Here's how the part is built. I have some questions about the finished solid (model axes, mm). Face numbers are marked on the shaded views. Give positions to 0.01 mm unless a question says otherwise; leave off trailing zeros. Write each loop counter-clockwise with the first axis right and the second up, starting at its lowest first coordinate (ties: lowest second). Pieces come first, ordered by that corner, then holes. Notation, with made-up numbers: M -38.5,23.25 L 4.5,23.25 A20 cw 4.5,41.25 Z; hole C 77.25,60.25 d7. An arc over 180 degrees is marked long. Answer as CSV lines item,"result". Start each with the question number.
Q1. Suppose I cut it at C-C (x = -790.5). Write out the boundary of the cut face in (y, z).
Q2. Suppose I cut it at B-B (z = 392). Write out the boundary of the cut face in (x, y).
Q3. If I drill on line 1 along Y through (x, z) = (55, 360.5); line 2 along Y through (x, z) = (481, 328.5); line 3 along X through (y, z) = (-389, 378.5), over which ranges is the centre line in solid material (lowest first)?
Q4. Thinking about a two-plate mould opening in Y: for the marked faces 1, 2, 3 and 4, which applies, +Y half, -Y half, draft (parallel to the pull), parting line (faces both ways), or undercut?
Q5. Suppose I cut it at A-A (y = 576). Write out the boundary of the cut face in (x, z), then the cut area to 3 significant figures.
Q6. For pin 1 (5 mm diameter, centred on x = -303.5, y = 399, fed in from +Z), with a flat end and sliding along its axis, tell me the tip position at first contact or that it passes through.
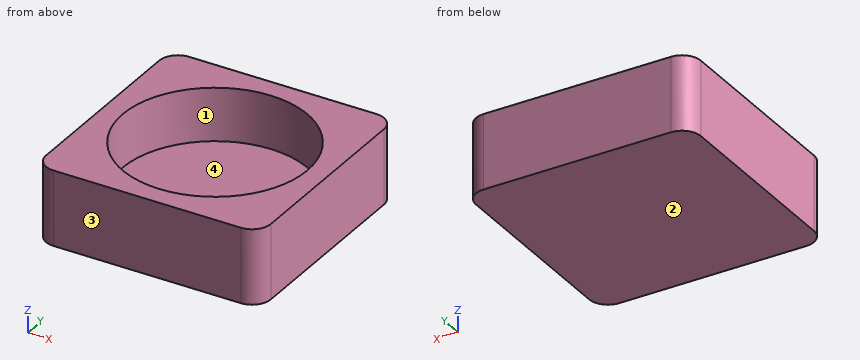
```python
from build123d import *

# Parameters (mm, degrees)
F0_W     = 1828.8
F0_H     = 1828.8
F1_DEPTH = 609.6
F2_R     = 751.405034
F3_DEPTH = 431.8
F4_R     = 152.4


with BuildPart() as f1:
    # F0 (on Top) → F1 (new body)
    with BuildSketch(Plane.XY):
        with Locations((-78.992321, -32.782064)):
            Rectangle(F0_W, F0_H)
    extrude(amount=F1_DEPTH)

    # F2 (on face) → F3 (cut)
    with BuildSketch(Plane.XY.offset(609.6)):
        with Locations((-78.992321, -32.782064)):
            Circle(F2_R)
    extrude(amount=-F3_DEPTH, mode=Mode.SUBTRACT)

    # F4
    f4_edges = [f1.edges().sort_by_distance(p)[0] for p in [
        (-993.392321, -947.182064, 304.8),
        (835.407679, -947.182064, 304.8),
        (835.407679, 881.617936, 304.8),
        (-993.392321, 881.617936, 304.8),
    ]]
    fillet(f4_edges, radius=F4_R)


solid = f1.part
```
Resolved:
1,outline,"M -947.18,0 L 881.62,0 L 881.62,609.6 L 208.81,609.6 L 208.81,177.8 L -274.37,177.8 L -274.37,609.6 L -947.18,609.6 Z"
2,outline,"M -993.39,-794.78 A152.4 ccw -840.99,-947.18 L 683.01,-947.18 A152.4 ccw 835.41,-794.78 L 835.41,729.22 A152.4 ccw 683.01,881.62 L -840.99,881.62 A152.4 ccw -993.39,729.22 Z; hole C -78.99,-32.78 d1502.81"
3,line 1,"-947.18 to -772.14, 706.58 to 881.62"
3,line 2,"-947.18 to -533.8, 468.24 to 881.62"
3,line 3,"-993.39 to -740.6, 582.61 to 835.41"
4,face 1,"undercut"
4,face 2,"draft"
4,face 3,"-Y half"
4,face 4,"undercut"
5,outline,"M -993.39,0 L 835.41,0 L 835.41,609.6 L 361.46,609.6 L 361.46,177.8 L -519.44,177.8 L -519.44,609.6 L -993.39,609.6 Z"
5,area,"734,000 mm^2"
6,pin 1,"z = 177.8"
